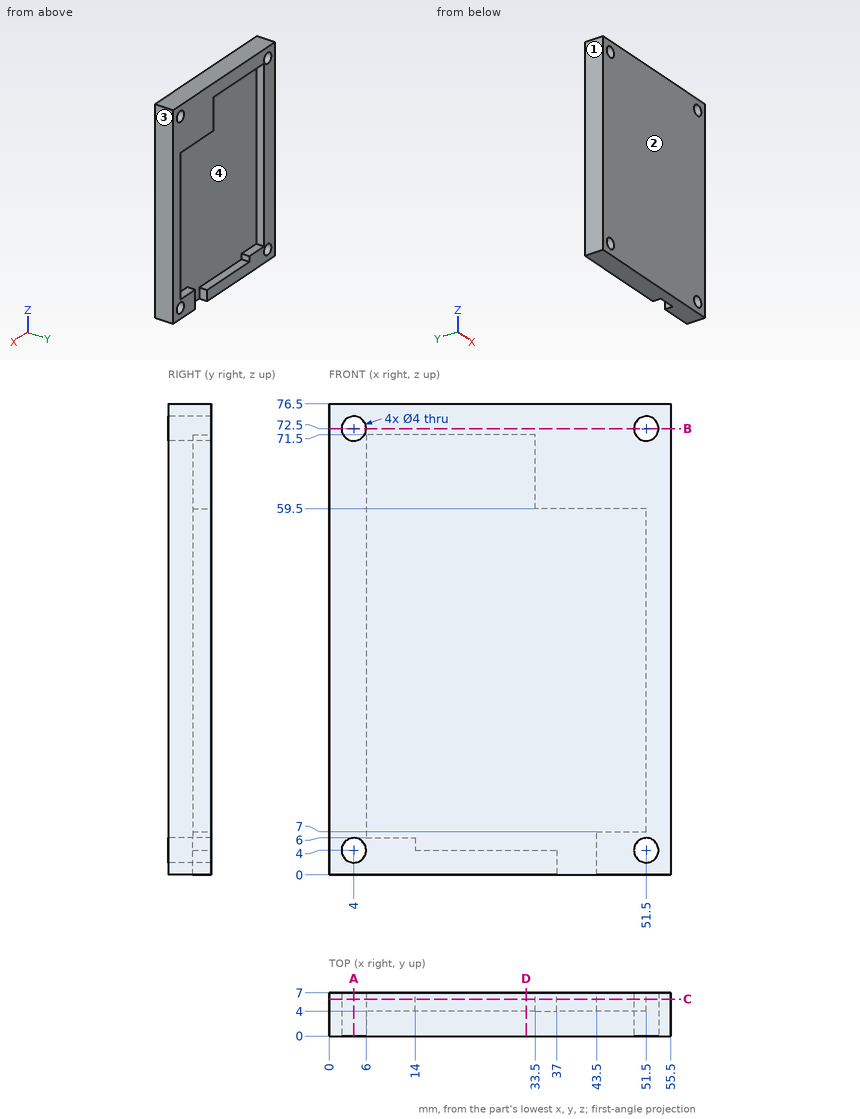
The drawing under review shows one solid part. Ordinate dimensions are in mm from its lowest x, y, z. Give positions to 0.01 mm unless a question says otherwise; leave off trailing zeros. Write each loop counter-clockwise with the first axis right and the second up, starting at its lowest first coordinate (ties: lowest second). Pieces come first, ordered by that corner, then holes. Notation, with made-up numbers: (70, 4) - (111, 4) arc R28 ccw to (111, 26) - close; hole circle Ø10 at (-6, -11.75). An arc over 180 degrees is marked (long way). Answer in a Markdown table with one row per item. Add a question column.
1. We need section B-B on z = 72.5. Write out the cut boundary in (x, y), then the cut area to 4 significant figures.
2. Wall thickness on line 1 along Z through (x, y) = (4, 2); line 2 along X through (y, z) = (2, 72.5); line 3 along Z through (x, y) = (19.5, 6): over which ranges is each line inside the solid? List them lowest first. Write a range as [from, to].
3. We need section D-D on x = 32. Write out the cut boundary in (y, z), then the cut area to 3 significant figures.
4. Insertion check: P1, Ø1.5, axis at x = 8, z = 14, coming from the +Y side; P2, Ø8, axis at x = 42, z = 69, coming from the -Y side; P3, Ø3.5, axis at x = 51.5, z = 72.5, coming from the +Y side. Each pin has a flat end and moves straight along its axis. Give the tip position at first contact, or say it passes through.
5. We need section C-C on y = 6. Write out the cut boundary in (x, z), then the cut area to 3 significant figures.
6. Draft analysis for pull direction X (two halves, no side actions). For the marked faces 1, 2, 3 and 4, state which applies: +X half, -X half, draft (parallel to the pull), parting line (faces both ways), or undercut.
7. We need section A-A on x = 4. Write out the cut boundary in (y, z), then the cut area to 4 significant figures.
Ans:
| question | item | result |
|---|---|---|
| 1 | outline | (0, 0) - (2, 0) - (2, 7) - (0, 7) - close; (6, 0) - (49.5, 0) - (49.5, 7) - (6, 7) - close; (53.5, 0) - (55.5, 0) - (55.5, 7) - (53.5, 7) - close |
| 1 | area | 332.5 mm^2 |
| 2 | line 1 | z = [0, 2], [6, 70.5], [74.5, 76.5] |
| 2 | line 2 | x = [0, 2], [6, 49.5], [53.5, 55.5] |
| 2 | line 3 | z = [0, 4], [71.5, 76.5] |
| 3 | outline | (0, 0) - (7, 0) - (7, 4) - (4, 4) - (4, 71.5) - (7, 71.5) - (7, 76.5) - (0, 76.5) - close |
| 3 | area | 333 mm^2 |
| 4 | P1 | stops at y = 4 |
| 4 | P2 | stops at y = 0 |
| 4 | P3 | passes through |
| 5 | outline | (0, 0) - (37, 0) - (37, 4) - (14, 4) - (14, 6) - (6, 6) - (6, 71.5) - (33.5, 71.5) - (33.5, 59.5) - (51.5, 59.5) - (51.5, 7) - (43.5, 7) - (43.5, 0) - (55.5, 0) - (55.5, 76.5) - (0, 76.5) - close; hole circle Ø4 at (4, 4); hole circle Ø4 at (4, 72.5); hole circle Ø4 at (51.5, 4); hole circle Ø4 at (51.5, 72.5) |
| 5 | area | 1,350 mm^2 |
| 6 | face 1 | -X half |
| 6 | face 2 | draft |
| 6 | face 3 | +X half |
| 6 | face 4 | undercut |
| 7 | outline | (0, 0) - (7, 0) - (7, 2) - (0, 2) - close; (0, 6) - (7, 6) - (7, 70.5) - (0, 70.5) - close; (0, 74.5) - (7, 74.5) - (7, 76.5) - (0, 76.5) - close |
| 7 | area | 479.5 mm^2 |
